from build123d import *

# Parameters (mm, degrees)
SKETCH_R  = 2.25
PAD_DEPTH = 1.5


with BuildPart() as part:
    # Sketch → Pad (new body)
    with BuildSketch(Plane.XY):
        with BuildLine():
            ThreePointArc((1.434501, 4.737584), (0, 4.95), (-1.434501, 4.737584))
            Line((-9.65, 2.25), (-1.434501, 4.737584))
            Line((-9.65, 2.25), (-9.65, -2.25))
            Line((-9.65, -2.25), (-1.434501, -4.737584))
            ThreePointArc((-1.434501, -4.737584), (0, -4.95), (1.434501, -4.737584))
            Line((1.434501, -4.737584), (9.65, -2.25))
            Line((9.65, 2.25), (9.65, -2.25))
            Line((1.434501, 4.737584), (9.65, 2.25))
        make_face()
        Circle(SKETCH_R, mode=Mode.SUBTRACT)
    extrude(amount=PAD_DEPTH)


solid = part.part
Read the model definition and answer for the solid it produces. Units are mm, in the model's axes. Coordinates: 2 decimals unless noted, no trailing zeros. Loops run counter-clockwise (first coordinate to the right, second up) from the corner with the lowest first, then second, coordinate; pieces in that order, holes last. Notation, with made-up numbers: (54.5, 77) -> (58.5, 77) arc R22 ccw to (58.5, 109) -> close; hole circle Ø2 at (-23, 38.5). An arc over 180 degrees is marked (long way). Answer in a Markdown table with one row per item.
Item 1: A cutting plane is placed at A-A on y = 0. Determine the outline of the cut face in (x, z), plus the area to 3 significant figures.
Returned:
| item | result |
|---|---|
| outline | (-9.65, 0) -> (-2.25, 0) -> (-2.25, 1.5) -> (-9.65, 1.5) -> close; (2.25, 0) -> (9.65, 0) -> (9.65, 1.5) -> (2.25, 1.5) -> close |
| area | 22.2 mm^2 |
Item 2: This flat-tipped pin is pushed along its axis until it touches: P1, Ø3.5, axis at x = 0, y = 0, coming from the +Z side. Where does it stop, or does it pass through?
Returned:
| item | result |
|---|---|
| P1 | passes through |
Item 3: A cutting plane is placed at C-C on z = 0.8. Determine the outline of the cut face in (x, y).
Returned:
| item | result |
|---|---|
| outline | (-9.65, -2.25) -> (-1.43, -4.74) arc R4.95 ccw to (1.43, -4.74) -> (9.65, -2.25) -> (9.65, 2.25) -> (1.43, 4.74) arc R4.95 ccw to (-1.43, 4.74) -> (-9.65, 2.25) -> close; hole circle Ø4.5 at (0, 0) |
Item 4: A cutting plane is placed at D-D on x = 7. Determine the outline of the cut face in (y, z).
Returned:
| item | result |
|---|---|
| outline | (-3.05, 0) -> (3.05, 0) -> (3.05, 1.5) -> (-3.05, 1.5) -> close |
Item 5: A cutting plane is placed at B-B on x = 0. Determine the outline of the cut face in (y, z).
Returned:
| item | result |
|---|---|
| outline | (-4.95, 0) -> (-2.25, 0) -> (-2.25, 1.5) -> (-4.95, 1.5) -> close; (2.25, 0) -> (4.95, 0) -> (4.95, 1.5) -> (2.25, 1.5) -> close |
Item 6: Straight lines are drawn through the part: line 1 along X through (y, z) = (1.25, 0.65); line 2 along X through (y, z) = (-0.5, 1.1); line 3 along Y through (x, z) = (-6.5, 0.8). For each, find the intervals that lie inside material, in ascending order. Write a range as [from, to].
Returned:
| item | result |
|---|---|
| line 1 | x = [-9.65, -1.87], [1.87, 9.65] |
| line 2 | x = [-9.65, -2.19], [2.19, 9.65] |
| line 3 | y = [-3.2, 3.2] |
Item 7: For a pull along X with two mould halves and no side action, classify faces 1 (the cylindrical face through (0.02, 4.95, 0.74)), 2 (the cylindrical face through (-0.29, 2.23, 0.74)), 3 (the flat face through (-9.65, 0, 1)) as released by +X, released by -X, zero draft, split by the parting line, or undercut.
Returned:
| item | result |
|---|---|
| face 1 | split by the parting line |
| face 2 | undercut |
| face 3 | released by -X |
